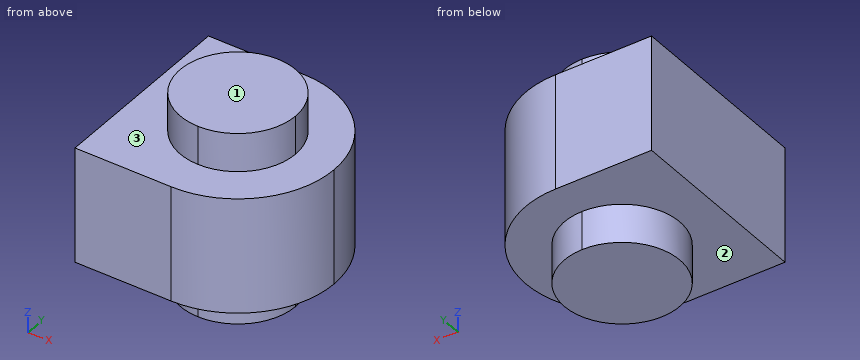
from build123d import *

# Parameters (mm, degrees)
F1_DEPTH = 7.62
F3_DEPTH = 2.54
F5_DEPTH = 2.54


with BuildPart() as f1:
    # F0 (on Top) → F1 (new body)
    with BuildSketch(Plane.XY):
        with BuildLine():
            ThreePointArc((-6.35, 6.35), (-4.4901280605, 1.8598719395), (0, 0))
            Line((0, 0), (0, 12.7))
            ThreePointArc((0, 12.7), (-4.4901280605, 10.8401280605), (-6.35, 6.35))
        make_face()
        with BuildLine():
            Line((0, 12.7), (0, 0))
            ThreePointArc((0, 0), (4.4901280605, 1.8598719395), (6.35, 6.35))
            ThreePointArc((6.35, 6.35), (4.4901280605, 10.8401280605), (0, 12.7))
        make_face()
        with BuildLine():
            Line((-6.35, 0), (0, 0))
            ThreePointArc((0, 0), (-4.4901280605, 1.8598719395), (-6.35, 6.35))
            Line((-6.35, 6.35), (-6.35, 0))
        make_face()
        with BuildLine():
            ThreePointArc((-6.35, 6.35), (-4.4901280605, 10.8401280605), (0, 12.7))
            Line((0, 12.7), (-6.35, 12.7))
            Line((-6.35, 12.7), (-6.35, 6.35))
        make_face()
    extrude(amount=F1_DEPTH)

    # F2 (on face) → F3 (join)
    with BuildSketch(Plane.XY.offset(7.62)):
        with BuildLine():
            ThreePointArc((0, 10.16), (-3.81, 6.35), (0, 2.54))
            Line((0, 2.54), (0, 10.16))
        make_face()
        with BuildLine():
            Line((0, 10.16), (0, 2.54))
            ThreePointArc((0, 2.54), (2.6940768363, 3.6559231637), (3.81, 6.35))
            ThreePointArc((3.81, 6.35), (2.6940768363, 9.0440768363), (0, 10.16))
        make_face()
    extrude(amount=F3_DEPTH)

    # F4 (on face) → F5 (join)
    with BuildSketch(Plane(origin=(0, 0, 0), x_dir=(1, 0, 0), z_dir=(0, 0, -1))):
        with BuildLine():
            ThreePointArc((0, -2.54), (-3.81, -6.35), (0, -10.16))
            Line((0, -10.16), (0, -2.54))
        make_face()
        with BuildLine():
            Line((0, -2.54), (0, -10.16))
            ThreePointArc((0, -10.16), (2.6940768363, -9.0440768363), (3.81, -6.35))
            ThreePointArc((3.81, -6.35), (2.6940768363, -3.6559231637), (0, -2.54))
        make_face()
    extrude(amount=F5_DEPTH)


solid = f1.part
Part model, mm, in its own coordinate system. Face numbers are marked on the shaded views. A direction names the side the tool comes from. Coordinates: 2 decimals unless noted, no trailing zeros. Order: outer loops, then holes, each group sorted by start corner. A loop starts at its lowest first (then second) coordinate and runs counter-clockwise, first axis right, second up. Notation, with made-up numbers: (57.5, 49.25) - (75.5, 49.25) arc R20 cw to (75.5, 73.25) - close; hole circle Ø10 at (-39.5, 51). An arc over 180 degrees is marked (long way). Use CSV: the item, a comma, the result in double quotes.
Item 1: Probe probe 1 along Z at (x, y) = (-4.25, 3); probe 2 along X at (y, z) = (3.5, -0.25); probe 3 along X at (y, z) = (3, 1). List the from-to ranges inside material, lowest first.
Solved:
probe 1,"z = 0 to 7.62"
probe 2,"x = -2.53 to 2.53"
probe 3,"x = -6.35 to 5.39"
Item 2: Saw through at C-C on y = 6. Give the cut face in (x, z).
Solved:
outline,"(-6.35, 0) - (-3.79, 0) - (-3.79, -2.54) - (3.79, -2.54) - (3.79, 0) - (6.34, 0) - (6.34, 7.62) - (3.79, 7.62) - (3.79, 10.16) - (-3.79, 10.16) - (-3.79, 7.62) - (-6.35, 7.62) - close"
Item 3: Saw through at A-A on z = 4. Give the cut face in (x, y), and give its area (3 significant figures).
Solved:
outline,"(-6.35, 0) - (0, 0) arc R6.35 ccw to (0, 12.7) - (-6.35, 12.7) - close"
area,"144 mm²"
Item 4: Saw through at B-B on x = -2.5. Give the cut face in (y, z).
Solved:
outline,"(0, 0) - (3.47, 0) - (3.47, -2.54) - (9.23, -2.54) - (9.23, 0) - (12.7, 0) - (12.7, 7.62) - (9.23, 7.62) - (9.23, 10.16) - (3.47, 10.16) - (3.47, 7.62) - (0, 7.62) - close"
Item 5: Saw through at D-D on x = 5.5. Give the cut face in (y, z).
Solved:
outline,"(3.18, 0) - (9.52, 0) - (9.52, 7.62) - (3.18, 7.62) - close"
Item 6: 3-axis set-ups, long thin cutter, end or side, ignore diameter. For the marked faces 1, 2 and 3: which of +Z, -Z, +X, -X, +Y, -Y reach the whole face in a straight line?
Solved:
face 1,"+Z, +X, -X, +Y, -Y"
face 2,"-Z"
face 3,"+Z"
Item 7: Drop flat-ended pins along their axis: P1, Ø2, axis at x = 2.5, y = 11.5, coming from the -Z side; P2, Ø5, axis at y = 8, z = 3, coming from the +X side; P3, Ø1.5, axis at y = 1.5, z = 5.5, coming from the +X side. Give the stop position or say it passes through.
Solved:
P1,"stops at z = 0"
P2,"stops at x = 6.35"
P3,"stops at x = 4.85"
